The drawing under review shows one solid part. Ordinate dimensions are in mm from its lowest x, y, z. A direction names the side the tool comes from. Coordinates: 2 decimals unless noted, no trailing zeros. Loops run counter-clockwise (first coordinate to the right, second up) from the corner with the lowest first, then second, coordinate; pieces in that order, holes last.
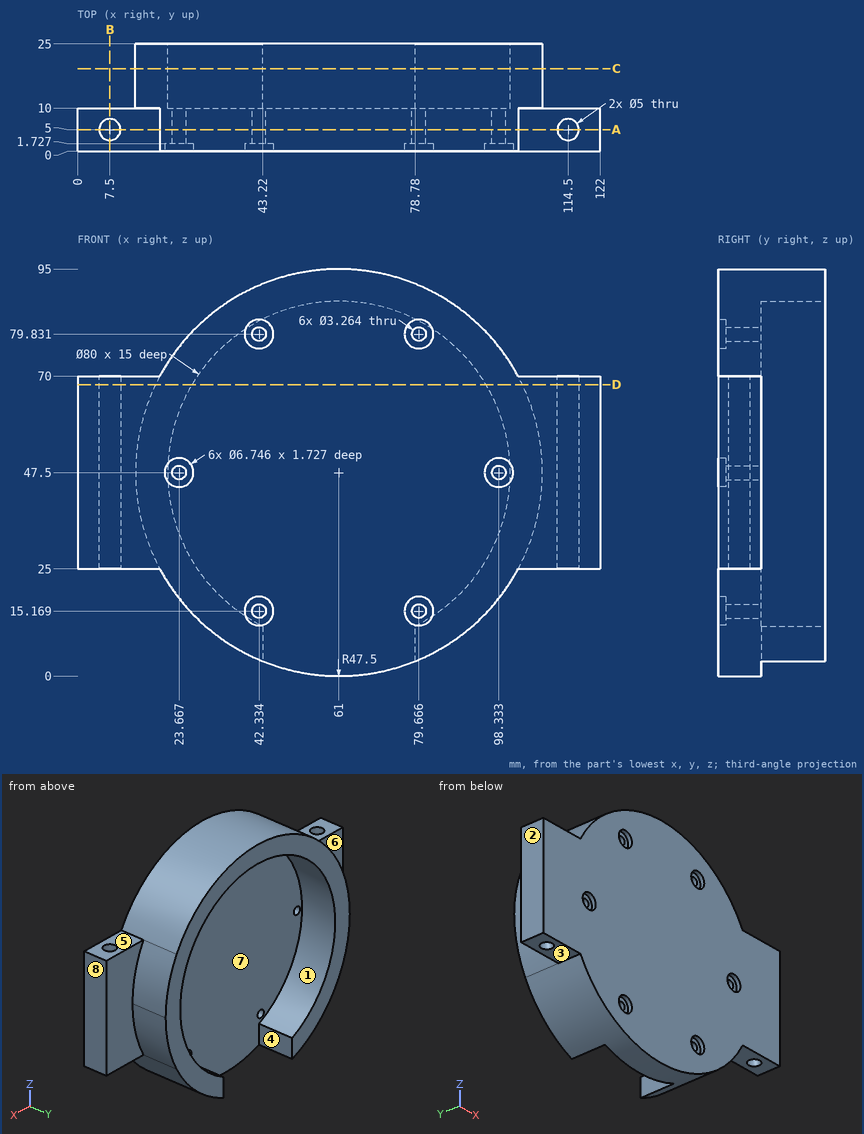
Q1. Machinability: for the marked faces 1, 2, 3, 4 and 5, which of the approach directions +Z, -Z, +X, -X, +Y, -Y give a long, thin tool a straight path to every point of the face, cutting with its end or side? Answer none if there is none.
Q2. Take a section at D-D, the plane z = 68. Write out the cut boundary in (x, y).
Q3. The part is to be moulded in two halves that separate along X. For the marked faces 6, 7 and 8, say which applies: pulls with the +X half, pulls with the -X half, needs draft (parallel to the pull), parting line crosses it, or undercut.
Q4. Take a section at B-B, the plane x = 7.5. Write out the cut boundary in (y, z).
Q5. Clearance check with flat-ended pins moving along their axes: pin 1 Ø6 at (y, z) = (9, 80) entering from +X; pin 2 Ø6 at (x, z) = (39, 77) entering from +Y; pin 3 Ø4 at (x, z) = (42.33, 15.17) entering from -Y. State where each tip first meets the part, or that it passes through.
Q6. Take a section at C-C, the plane y = 19.25. Write out the cut boundary in (x, z), then the cut area to 3 significant figures.
Q7. For line 1 (Y direction, x = 7.5, z = 46.5); line 2 (X direction, y = 6.75, z = 47.5) (1 decimal); line 3 (X direction, y = 16, z = 39) (1 decimal), list the stretches that pass through material, from the lowest coordinate up.
Q8. Take a section at A-A, the plane y = 5. Give the number of separate pieces and of enclosed holes in the cut face, then the cut area to 3 significant figures.
Entries:
1. face 1: +Y
1. face 2: +Z, -Z, -X, +Y, -Y
1. face 3: -Z, -X, +Y, -Y
1. face 4: -Z, +Y
1. face 5: +Z, +X, +Y, -Y
2. outline: (0, 0) - (122, 0) - (122, 10) - (103.85, 10) - (103.85, 25) - (95.35, 25) - (95.35, 10) - (26.65, 10) - (26.65, 25) - (18.15, 25) - (18.15, 10) - (0, 10) - close; hole circle Ø5 at (7.5, 5); hole circle Ø5 at (114.5, 5)
3. face 6: needs draft
3. face 7: undercut
3. face 8: pulls with the +X half
4. outline: (0, 25) - (2.5, 25) - (2.5, 70) - (0, 70) - close; (7.5, 25) - (10, 25) - (10, 70) - (7.5, 70) - close
5. pin 1: stops at x = 98.23
5. pin 2: stops at y = 10
5. pin 3: stops at y = 1.73
6. outline: (43.22, 3.45) - (43.22, 11.67) arc R40 cw (long way) to (78.78, 11.67) - (78.78, 3.45) arc R47.5 ccw (long way) to start
6. area: 1,790 mm2
7. line 1: y = 0 to 2.5, 7.5 to 10
7. line 2: x = 0 to 5.7, 9.3 to 22, 25.3 to 96.7, 100 to 112.7, 116.3 to 122
7. line 3: x = 14.3 to 21.9, 100.1 to 107.7
8. separate pieces: 3
8. enclosed holes: 6
8. area: 7,970 mm2
